Read the model definition and answer for the solid it produces. Units are mm, in the model's axes. A direction names the side the tool comes from. Give positions to 0.01 mm unless a question says otherwise; leave off trailing zeros. Write each loop counter-clockwise with the first axis right and the second up, starting at its lowest first coordinate (ties: lowest second). Pieces come first, ordered by that corner, then holes.
```python
from build123d import *

# Parameters (mm, degrees)
BOSS_EXTRUDE1_START = 20.333687
BOSS_EXTRUDE1_DEPTH = 11.1125


with BuildPart() as part:
    # Sketch1 → Boss-Extrude1 (new body)
    with BuildSketch(Plane.XY.offset(BOSS_EXTRUDE1_START)):
        Polygon((293.574186737, -297.8658), (293.574186737, -310.5658), (99.899186737, -310.5658), (99.899186737, -297.8658), (99.899186737, -25.8475), (293.574186737, -25.8475), align=None)
        with BuildLine():
            ThreePointArc((250.711686737, -151.555275), (245.076061737, -157.1909), (250.711686737, -162.826525))
            Line((250.711686737, -162.826525), (276.111686737, -162.826525))
            ThreePointArc((276.111686737, -162.826525), (281.747311737, -157.1909), (276.111686737, -151.555275))
            Line((276.111686737, -151.555275), (250.711686737, -151.555275))
        make_face(mode=Mode.SUBTRACT)
        with BuildLine():
            ThreePointArc((250.711686737, -81.705275), (245.076061737, -87.3409), (250.711686737, -92.976525))
            Line((250.711686737, -92.976525), (276.111686737, -92.976525))
            ThreePointArc((276.111686737, -92.976525), (281.747311737, -87.3409), (276.111686737, -81.705275))
            Line((276.111686737, -81.705275), (250.711686737, -81.705275))
        make_face(mode=Mode.SUBTRACT)
        with BuildLine():
            ThreePointArc((168.161686737, -92.976525), (173.797311737, -87.3409), (168.161686737, -81.705275))
            Line((168.161686737, -81.705275), (142.761686737, -81.705275))
            ThreePointArc((142.761686737, -81.705275), (137.126061737, -87.3409), (142.761686737, -92.976525))
            Line((142.761686737, -92.976525), (168.161686737, -92.976525))
        make_face(mode=Mode.SUBTRACT)
        with BuildLine():
            ThreePointArc((142.761686737, -151.555275), (137.126061737, -157.1909), (142.761686737, -162.826525))
            Line((142.761686737, -162.826525), (168.161686737, -162.826525))
            ThreePointArc((168.161686737, -162.826525), (173.797311737, -157.1909), (168.161686737, -151.555275))
            Line((168.161686737, -151.555275), (142.761686737, -151.555275))
        make_face(mode=Mode.SUBTRACT)
    extrude(amount=BOSS_EXTRUDE1_DEPTH)


solid = part.part
```
Item 1: Determine the mould class of faces 3 (the flat face through (293.574, -170, 26)), 4 (the flat face through (198, -166, 31.446)), 5 (the flat face through (264, -81.705, 26)), 6 (the flat face through (99.899, -166, 26)) for opening direction X: pulls with the +X half, pulls with the -X half, needs draft (parallel to the pull), parting line crosses it, or undercut.
Result set:
face 3: pulls with the +X half
face 4: needs draft
face 5: undercut
face 6: pulls with the -X half
Item 2: Section B-B (z = 27.75) is taken. Write down the section's boundary in (x, y), and give its area (3 significant figures).
Result set:
outline: (99.9, -310.57) - (293.57, -310.57) - (293.57, -25.85) - (99.9, -25.85) - close; hole (142.76, -162.83) - (168.16, -162.83) arc R5.64 ccw to (168.16, -151.56) - (142.76, -151.56) arc R5.64 ccw to start; hole (142.76, -92.98) - (168.16, -92.98) arc R5.64 ccw to (168.16, -81.71) - (142.76, -81.71) arc R5.64 ccw to start; hole (250.71, -162.83) - (276.11, -162.83) arc R5.64 ccw to (276.11, -151.56) - (250.71, -151.56) arc R5.64 ccw to start; hole (250.71, -92.98) - (276.11, -92.98) arc R5.64 ccw to (276.11, -81.71) - (250.71, -81.71) arc R5.64 ccw to start
area: 53,600 mm2
Item 3: Find the intervals of material crossed by line 1 along Y through (x, z) = (145, 27.5), in increasing order.
Result set:
line 1: y = -310.57 to -162.83, -151.56 to -92.98, -81.71 to -25.85
Item 4: Which of the six approach directions +Z, -Z, +X, -X, +Y, -Y give full straight-line access (tool end or side, diameter ignored) to faces 1 (the cylindrical face through (173.796, -157.315, 25.812)), 2 (the flat face through (198, -310.566, 26))?
Result set:
face 1: +Z, -Z
face 2: +Z, -Z, +X, -X, -Y
Item 5: Section A-A (x = 158) is taken. Write down the section's boundary in (y, z).
Result set:
outline: (-310.57, 20.33) - (-162.83, 20.33) - (-162.83, 31.45) - (-310.57, 31.45) - close; (-151.56, 20.33) - (-92.98, 20.33) - (-92.98, 31.45) - (-151.56, 31.45) - close; (-81.71, 20.33) - (-25.85, 20.33) - (-25.85, 31.45) - (-81.71, 31.45) - close
